Study the drawing (mm; zero at the part's minimum x, y, z) and answer. Coordinates: 2 decimals unless noted, no trailing zeros. Loops run counter-clockwise (first coordinate to the right, second up) from the corner with the lowest first, then second, coordinate; pieces in that order, holes last. Notation, with made-up numbers: (71.5, 0) - (123.5, 0) arc R18 cw to (123.5, 8) - close; hole circle Ø6 at (16, 75). An arc over 180 degrees is marked (long way). Put each result on its own line as item: value.
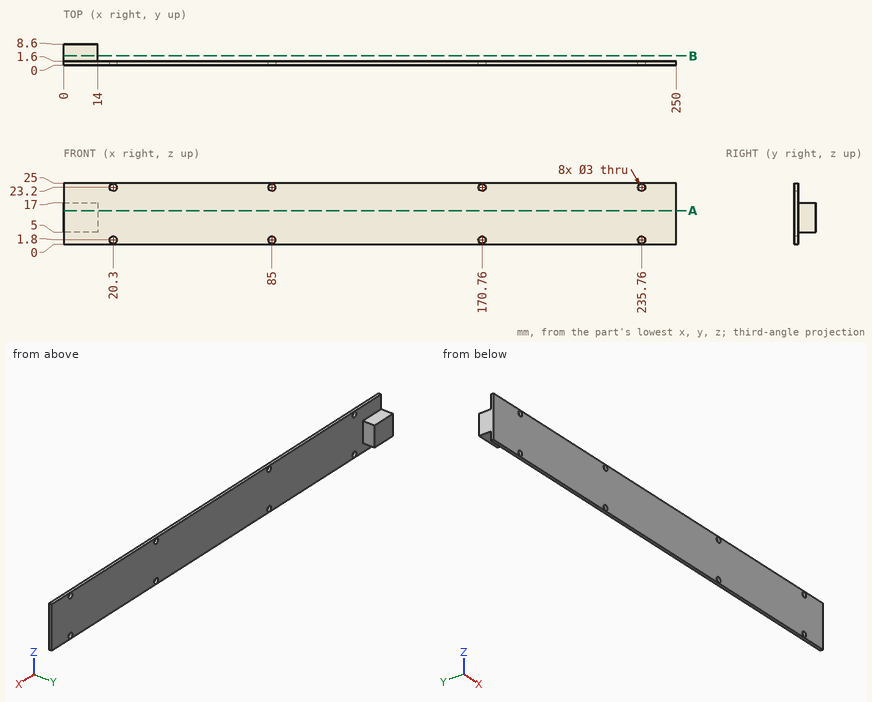
1) The part is cut by section A-A (z = 13.75). Give the vertices of the cut face in (x, y).
Found:
outline: (0, 0) - (250, 0) - (250, 1.6) - (14, 1.6) - (14, 8.6) - (0, 8.6) - close
2) Straight lines are drawn through the part: L1, parallel to Z at x = 235.76, y = 0.85; L2, parallel to Y at x = 113, z = 21.25. For each, find the intervals that lie inside material, in ascending order. Write a range as [from, to].
Found:
L1: z = [0, 0.3], [3.3, 21.7], [24.7, 25]
L2: y = [0, 1.6]
3) The part is cut by section B-B (y = 3.75). Give the vertices of the cut face in (x, z), and give its area (3 significant figures).
Found:
outline: (0, 5) - (14, 5) - (14, 17) - (0, 17) - close
area: 168 mm^2
4) Each of these flat-tipped pins is pushed along its axis until it touches: pin 1 (2 mm diameter, centred on y = 4.5, z = 13.5, fed in from +X); pin 2 (2 mm diameter, centred on x = 5, y = 7, fed in from +Z); pin 3 (5 mm diameter, centred on y = 5, z = 22.5, fed in from -X); pin 4 (3.5 mm diameter, centred on x = 85, z = 23.2, fed in from +Y). Where does it stop, or does it pass through?
Found:
pin 1: stops at x = 14
pin 2: stops at z = 17
pin 3: passes through
pin 4: stops at y = 1.6
